```python
from build123d import *

# Parameters (mm, degrees)
SKETCH1_W             = 63
SKETCH1_H             = 55
BOSS_EXTRUDE1_DEPTH   = 45
SHELL1_T              = -5
SKETCH5_W             = 20
SKETCH5_H             = 8
SKETCH5_W_2           = 6.3754
SKETCH5_H_2           = 20
SKETCH5_W_3           = 6.35
BOSS_EXTRUDE3_DEPTH   = 5
F_6_CLEARANCE_HOLE1_D = 3.7973


with BuildPart() as part:
    # Sketch1 → Boss-Extrude1 (new body)
    with BuildSketch(Plane(origin=(0, 0, 0), x_dir=(1, 0, 0), z_dir=(0, 1, 0))):
        with Locations((-11.452841564, -4.099064972)):
            Rectangle(SKETCH1_W, SKETCH1_H)
    extrude(amount=BOSS_EXTRUDE1_DEPTH)

    # Shell1
    shell1_openings = [part.faces().sort_by_distance(p)[0] for p in [
        (-11.452841564, 45, 4.099064972),
    ]]
    offset(amount=SHELL1_T, openings=shell1_openings, kind=Kind.INTERSECTION)

    # Sketch5 → Boss-Extrude3 (add)
    with BuildSketch(Plane(origin=(0, 45, 0), x_dir=(1, 0, 0), z_dir=(0, 1, 0))):
        with Locations((-11.452841564, 27.400935028)):
            Rectangle(SKETCH5_W, SKETCH5_H)
        with Locations((-11.452841564, -35.599064972)):
            Rectangle(SKETCH5_W, SKETCH5_H)
        with Locations((-46.140541564, -4.099064972)):
            Rectangle(SKETCH5_W_2, SKETCH5_H_2)
        with Locations((23.222158436, -4.099064972)):
            Rectangle(SKETCH5_W_3, SKETCH5_H_2)
    extrude(amount=-BOSS_EXTRUDE3_DEPTH)

    # #6 Clearance Hole1 (through all)
    with Locations(Plane(origin=(0, 40, 0), x_dir=(-1, 0, 0), z_dir=(0, -1, 0))):
        with Locations((11.452841564, -35.599064972), (11.452841564, 27.400935028), (46.140541564, -4.099064972), (-23.222158436, -4.099064972)):
            Hole(F_6_CLEARANCE_HOLE1_D / 2)


solid = part.part
```
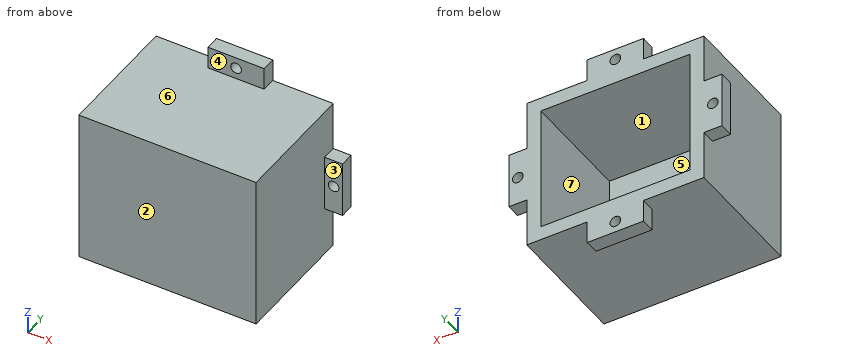
Can you work these out from the model? Positions are in its coordinate system, mm. Face numbers are marked on the shaded views. A direction names the side the tool comes from. Give positions to 0.01 mm unless a question says otherwise; leave off trailing zeros. Write each loop counter-clockwise with the first axis right and the second up, starting at its lowest first coordinate (ties: lowest second). Pieces come first, ordered by that corner, then holes. Notation, with made-up numbers: (-34, -11) -> (-10, -11) arc R27 cw to (-10, 5) -> close; hole circle Ø6 at (51, -24.5). An arc over 180 degrees is marked (long way). Write item = value, one per line.
(1) I need wall thicknesses on probe 1 along X at (y, z) = (35, -2); probe 2 along Z at (x, y) = (-3, 19); probe 3 along Y at (x, z) = (-10, -8). Which ranges of each line are inside material? Lowest first, please. Write a range as from..to.
Worked out:
probe_1 = -42.95..-37.95, 15.05..20.05
probe_2 = -23.4..-18.4, 26.6..31.6
probe_3 = 0..5
(2) Suppose I cut it at C-C on y = 6. Write out the boundary of the cut face in (x, z), then the cut area to 3 significant figures.
Worked out:
outline = (-42.95, -23.4) -> (20.05, -23.4) -> (20.05, 31.6) -> (-42.95, 31.6) -> close; hole (-37.95, -18.4) -> (15.05, -18.4) -> (15.05, 26.6) -> (-37.95, 26.6) -> close
area = 1,080 mm^2
(3) Suppose I cut it at B-B on z = -15. Write out the boundary of the cut face in (x, y), then the cut area to 3 significant figures.
Worked out:
outline = (-42.95, 0) -> (20.05, 0) -> (20.05, 45) -> (15.05, 45) -> (15.05, 5) -> (-37.95, 5) -> (-37.95, 45) -> (-42.95, 45) -> close
area = 715 mm^2
(4) Suppose I cut it at A-A on x = -5.5. Write out the boundary of the cut face in (y, z), then the cut area to 3 significant figures.
Worked out:
outline = (0, -23.4) -> (40, -23.4) -> (40, -31.4) -> (45, -31.4) -> (45, -18.4) -> (5, -18.4) -> (5, 26.6) -> (45, 26.6) -> (45, 39.6) -> (40, 39.6) -> (40, 31.6) -> (0, 31.6) -> close
area = 755 mm^2
(5) Thinking about a two-plate mould opening in X: for the marked faces 5, 6 and 7, which applies, released by +X, released by -X, zero draft, split by the parting line, or undercut?
Worked out:
face_5 = undercut
face_6 = zero draft
face_7 = undercut
(6) Suppose I cut it at D-D on z = -0.5. Write out the boundary of the cut face in (x, y).
Worked out:
outline = (-49.33, 40) -> (-42.95, 40) -> (-42.95, 0) -> (20.05, 0) -> (20.05, 40) -> (26.4, 40) -> (26.4, 45) -> (15.05, 45) -> (15.05, 5) -> (-37.95, 5) -> (-37.95, 45) -> (-49.33, 45) -> close
(7) I'm going to push flat-ended pins straight in: P1, Ø3, axis at x = 23.22, z = 4.1, coming from the -Y side; P2, Ø22.5, axis at x = -15, y = 16.5, coming from the -Z side; P3, Ø1.5, axis at y = 42, z = -26.5, coming from the +X side; P4, Ø8, axis at x = -33.5, z = 18, coming from the +Y side. Where does each tip first touch, or does it pass through?
Worked out:
P1 = through
P2 = -23.4
P3 = -1.45
P4 = 5
(8) For the marked faces 1, 2, 3 and 4, which set-ups out of +Z, -Z, +X, -X, +Y, -Y let a thin tool reach every point of the face, with its end or its side?
Worked out:
face_1 = +Y
face_2 = +Z, -Z, +X, -X, -Y
face_3 = +Z, -Z, +X, -Y
face_4 = +Z, +X, -X, -Y
